Autodesk Inventor part; units mm, degrees
ref_plane "YZ Plane" through (0, 0, 0) normal (1, 0, 0) x (0, 1, 0)
ref_plane "XZ Plane" through (0, 0, 0) normal (0, 1, 0) x (-1, 0, 0)
ref_plane "XY Plane" through (0, 0, 0) normal (0, 0, 1) x (1, 0, 0)
sketch "Sketch1" plane through (0, 0, 0) normal (0, 0, 1) x (1, 0, 0)
  line L0 (19.7536, 18.501) -> (19.7536, -51.499)
  line L1 (-40.2464, -51.499) -> (-40.2464, 18.501)
  line L2 (-40.2464, -51.499) -> (-30.2464, -61.499)
  line L3 (-30.2464, -61.499) -> (9.7536, -61.499)
  line L4 (9.7536, -61.499) -> (19.7536, -51.499)
  line L5 (5.9033, -42.3953) -> (-35.9604, 24.6005)
  line L6 (-41.4722, 25.873) -> (-55.041, 17.3943)
  line L7 (-60.5529, 18.6668) -> (-71.151, 35.6275)
  line L8 (8.6592, -43.0315) -> (13.7475, -39.852)
  line L9 (14.3837, -37.0961) -> (-27.4799, 29.8997)
  line L10 (-26.2074, 35.4116) -> (-14.9119, 42.4698)
  line L11 (-15.0424, 49.3323) -> (-34.727, 60.6155)
  line L12 (-38.8359, 60.5374) -> (-69.8786, 41.1398)
  arc A0 (-34.727, 60.6155) -> (-38.8359, 60.5374) centre (-36.7162, 57.1452) ccw
  arc A1 (-14.9119, 42.4698) -> (-15.0424, 49.3323) centre (-17.0316, 45.8619) ccw
  arc A2 (-35.9604, 24.6005) -> (-41.4722, 25.873) centre (-39.3526, 22.4808) ccw
  arc A3 (-26.2074, 35.4116) -> (-27.4799, 29.8997) centre (-24.0877, 32.0194) ccw
  arc A4 (5.9033, -42.3953) -> (8.6592, -43.0315) centre (7.5994, -41.3354) ccw
  arc A5 (13.7475, -39.852) -> (14.3837, -37.0961) centre (12.6876, -38.1559) ccw
  line L13 (-26.3961, -42.3953) -> (15.4675, 24.6005)
  line L14 (20.9794, 25.873) -> (34.5482, 17.3943)
  line L15 (40.3411, 19.095) -> (50.6682, 35.6217)
  line L16 (-29.152, -43.0315) -> (-34.2403, -39.852)
  line L17 (-34.8766, -37.0961) -> (6.9871, 29.8997)
  line L18 (5.7136, 35.4098) -> (-5.5789, 42.4725)
  line L19 (-5.4504, 49.3323) -> (14.2435, 60.6103)
  line L20 (18.3431, 60.5374) -> (49.3859, 41.1397)
  arc A6 (18.3431, 60.5374) -> (14.2435, 60.6103) centre (16.2322, 57.1397) ccw
  arc A7 (-5.4504, 49.3323) -> (-5.5789, 42.4725) centre (-3.4579, 45.8638) ccw
  arc A8 (20.9794, 25.873) -> (15.4675, 24.6005) centre (18.8597, 22.4808) ccw
  arc A9 (6.9871, 29.8997) -> (5.7136, 35.4098) centre (3.5938, 32.0177) ccw
  arc A10 (-29.152, -43.0315) -> (-26.3961, -42.3953) centre (-28.0922, -41.3354) ccw
  arc A11 (-34.8766, -37.0961) -> (-34.2403, -39.852) centre (-33.1805, -38.1559) ccw
  arc A12 (-15.0424, 49.3323) -> (-5.4504, 49.3323) centre (-10.2464, 55.8144) ccw
  circle A13 centre (-10.2464, -7.115) radius 26
  circle A14 centre (-10.2464, -7.115) radius 20
  line L21 (-40.2464, 18.501) -> (-40.2464, 26.3797)
  line L22 (19.7536, 18.501) -> (19.7536, 26.3797)
  line L23 (-60.5529, 18.6668) -> (-60.5529, 18.6668)
  line L24 (-55.041, 17.3943) -> (-55.041, 17.3943)
  line L25 (-69.8786, 41.1398) -> (-69.8787, 41.1397)
  line L26 (-71.1513, 35.6278) -> (-71.151, 35.6275)
  arc A15 (-69.8787, 41.1397) -> (-71.1513, 35.6278) centre (-67.7591, 37.7475) ccw
  arc A16 (-60.5529, 18.6668) -> (-55.041, 17.3943) centre (-57.1607, 20.7865) ccw
  line L27 (49.3957, 41.1336) -> (49.3859, 41.1397)
  line L28 (50.6682, 35.6217) -> (50.6682, 35.6217)
  line L29 (34.5482, 17.3943) -> (34.5579, 17.3883)
  line L30 (40.3411, 19.095) -> (40.0698, 18.6608)
  arc A17 (34.5579, 17.3883) -> (40.0698, 18.6608) centre (36.6776, 20.7804) ccw
  arc A18 (50.6682, 35.6217) -> (49.3957, 41.1336) centre (47.276, 37.7414) ccw
  point P0 (0, 0)
  point P1 (-9.2464, 46.01)
  point P2 (-36.8049, 61.8065)
  point P3 (-20.4928, 0)
  point P4 (-11.243, 46.015)
  point P5 (16.3218, 61.8004)
  dimension "d0" = 70
  dimension "d1" = 135
  dimension "d2" = 135
  dimension "d3" = 10
  dimension "d4" = 10
  dimension "d5" = 40
  dimension "d6" = 10
  dimension "d7" = 85
  dimension "d8" = 24
  dimension "d9" = 24
  dimension "d10" = 28
  dimension "d11" = 43
  dimension "d13" = 2
  dimension "d14" = 31
  dimension "d15" = 32
  dimension "d19" = 70
  dimension "d21" = 52
  dimension "d22" = 40
  dimension "d43" = 8.0635
  dimension "d66" = 54.384
  dimension "d74" = 4
  dimension "d75" = 4
  dimension "d77" = 43
  dimension "d78" = 85
  dimension "d79" = 4
extrude "Extrusion2" add sketch "Sketch1" along normal blind 1
sketch "Sketch11" plane through (0, 0, 1) normal (0, 0, 1) x (1, 0, 0)
  line L0 (40.0698, 18.6608) -> (50.6682, 35.6217)
  line L1 (-15.0424, 49.3323) -> (-34.727, 60.6155)
  arc A0 (-34.727, 60.6155) -> (-38.8359, 60.5374) centre (-36.7162, 57.1452) ccw
  line L2 (-38.8359, 60.5374) -> (-69.8787, 41.1397)
  arc A1 (-69.8787, 41.1397) -> (-71.1513, 35.6278) centre (-67.7591, 37.7475) ccw
  line L3 (-71.1513, 35.6278) -> (-60.5529, 18.6668)
  arc A2 (-60.5529, 18.6668) -> (-55.041, 17.3943) centre (-57.1607, 20.7865) ccw
  line L4 (-55.041, 17.3943) -> (-41.4722, 25.873)
  arc A3 (-40.2464, 26.3797) -> (-41.4722, 25.873) centre (-39.3526, 22.4808) ccw
  line L5 (-40.2464, 26.3797) -> (-40.2464, -51.499)
  line L6 (-40.2464, -51.499) -> (-30.2464, -61.499)
  line L7 (-30.2464, -61.499) -> (9.7536, -61.499)
  line L8 (9.7536, -61.499) -> (19.7536, -51.499)
  line L9 (19.7536, -51.499) -> (19.7536, 26.3797)
  arc A4 (20.9794, 25.873) -> (19.7536, 26.3797) centre (18.8597, 22.4808) ccw
  line L10 (20.9794, 25.873) -> (34.5579, 17.3883)
  arc A5 (34.5579, 17.3883) -> (40.0698, 18.6608) centre (36.6776, 20.7804) ccw
  line L11 (40.0698, 18.6608) -> (50.6682, 35.6217)
  arc A6 (50.6682, 35.6217) -> (49.3957, 41.1336) centre (47.276, 37.7414) ccw
  line L12 (49.3957, 41.1336) -> (18.3431, 60.5374)
  arc A7 (18.3431, 60.5374) -> (14.2435, 60.6103) centre (16.2322, 57.1397) ccw
  line L13 (14.2435, 60.6103) -> (-5.4504, 49.3323)
  arc A8 (-5.4504, 49.3323) -> (-5.9605, 48.9843) centre (-3.4579, 45.8638) ccw
  arc A9 (-14.528, 48.9816) -> (-5.9605, 48.9843) centre (-10.2464, 55.8144) ccw
  arc A10 (-14.528, 48.9816) -> (-15.0424, 49.3323) centre (-17.0316, 45.8619) ccw
  line L14 (41.5088, 46.0618) -> (26.6711, 22.3165)
  point P0 (0, 0)
  dimension "d80" = 13.3
extrude "Extrusion9" cut sketch "Sketch11" against normal blind 10 contours A5 L10 L14 L12 A6 L0
properties part number "Boilermake_PCBMechanicalOverlay"
Read the model definition and answer for the solid it produces. Units are mm, in the model's axes. A direction names the side the tool comes from. Coordinates: 2 decimals unless noted, no trailing zeros. Loops run counter-clockwise (first coordinate to the right, second up) from the corner with the lowest first, then second, coordinate; pieces in that order, holes last.
(1) The part is cut by section D-D (y = 11). Determine the outline of the cut face in (x, z).
Solution:
outline: (-40.25, 0) - (19.75, 0) - (19.75, 1) - (-40.25, 1) - close
(2) A flat-ended cylindrical pin translates along its axis: pin 1 Ø0.5 at (y, z) = (-16.5, 0.5) entering from +X. Find the tip coordinate at first contact, or state that the pin passes through.
Solution:
pin 1: stops at x = 19.75
(3) The mould has two halves that part along X. Classify faces 1 (the face through (-16, 14, 0)), 2 (the face through (23.785, 24.12, 0.493)), 3 (the face through (-65.78, 27.03, 0.49)), 4 (the face through (-48.162, 21.693, 0.493)): released by +X, released by -X, zero draft, split by the parting line, or undercut.
Solution:
face 1: zero draft
face 2: undercut
face 3: released by -X
face 4: undercut
(4) The part is cut by section B-B (z = 0.65). Determine the outline of the cut face in (x, y).
Solution:
outline: (-71.15, 35.63) - (-60.55, 18.67) arc R4 ccw to (-55.04, 17.39) - (-41.47, 25.87) arc R4 cw to (-40.25, 26.38) - (-40.25, -51.5) - (-30.25, -61.5) - (9.75, -61.5) - (19.75, -51.5) - (19.75, 26.38) arc R4 cw to (20.98, 25.87) - (26.67, 22.32) - (41.51, 46.06) - (18.34, 60.54) arc R4 ccw to (14.24, 60.61) - (-5.45, 49.33) arc R4 ccw to (-5.96, 48.98) arc R8.06 cw to (-14.53, 48.98) arc R4 ccw to (-15.04, 49.33) - (-34.73, 60.62) arc R4 ccw to (-38.84, 60.54) - (-69.88, 41.14) arc R4 ccw to start
(5) The part is cut by section C-C (x = -44). Determine the outline of the cut face in (y, z), and give its area (3 significant figures).
Solution:
outline: (24.29, 0) - (57.31, 0) - (57.31, 1) - (24.29, 1) - close
area: 33.0 mm2
(6) Consider line 1 along X through (y, z) = (22.5, 0.9); line 2 along X through (y, z) = (-24.5, 0.9); line 3 along Y through (x, z) = (-62, 0.8). Determine where each line is inside the solid, lowest interval first.
Solution:
line 1: x = -62.95 to -46.87, -40.25 to 19.75, 26.38 to 26.79
line 2: x = -40.25 to 19.75
line 3: y = 20.98 to 46.06
(7) The part is cut by section A-A (y = 52.5). Determine the outline of the cut face in (x, z), and give its area (3 significant figures).
Solution:
outline: (-51.7, 0) - (-20.57, 0) - (-20.57, 1) - (-51.7, 1) - close; (0.08, 0) - (31.21, 0) - (31.21, 1) - (0.08, 1) - close
area: 62.3 mm2
(8) A tool of negligible diameter and unlimited length cuts with its end or side. For faces 5 (the face through (4.259, 54.892, 0.493)), 6 (the face through (34.194, 34.355, 0.507)), from which of +Z, -Z, +X, -X, +Y, -Y can it reach the whole face along a straight path? Write none if from no direction.
Solution:
face 5: +Z, -Z, +Y
face 6: +Z, -Z, +X, -Y
